from build123d import *

# Parameters (mm, degrees)
BOSS_EXTRUDE1_DEPTH     = 2
SKETCH2_R               = 3.25
CUT_HOLES_DEPTH         = 3
CUT_HOLES_DEPTH_BACK    = 3
CUT_EXTRUDE1_DEPTH      = 3
CUT_EXTRUDE1_DEPTH_BACK = 3


with BuildPart() as part:
    # Sketch1 → Boss-Extrude1 (new body, symmetric)
    with BuildSketch(Plane(origin=(0, 0, 0), x_dir=(1, 0, 0), z_dir=(0, 1, 0))):
        with BuildLine():
            Line((86.2, 39.931942102), (86.2, -39.931942102))
            ThreePointArc((86.2, -39.931942102), (0, -81.597763245), (-86.2, -39.931942102))
            Line((-86.2, -39.931942102), (-86.2, 39.931942102))
            ThreePointArc((-86.2, 39.931942102), (0, 95), (86.2, 39.931942102))
        make_face()
    extrude(amount=BOSS_EXTRUDE1_DEPTH, both=True)

    # Sketch2 → Cut-Holes (cut, two sides)
    with BuildSketch(Plane(origin=(0, 0, 0), x_dir=(1, 0, 0), z_dir=(0, 1, 0))) as cut_holes_sk:
        with Locations((-74.7, 11)):
            Circle(SKETCH2_R)
        with Locations((-74.7, -41)):
            Circle(SKETCH2_R)
        with Locations((74.7, -41)):
            Circle(SKETCH2_R)
        with Locations((74.7, 11)):
            Circle(SKETCH2_R)
        with Locations((0, -71.597763245)):
            Circle(SKETCH2_R)
        with Locations((0, 85)):
            Circle(SKETCH2_R)
        with Locations((-75.036257902, 39.931942102)):
            Circle(SKETCH2_R)
        with Locations((75.036257902, 39.931942102)):
            Circle(SKETCH2_R)
        with BuildLine():
            ThreePointArc((14.471626034, -67.259325745), (11.744315506, -70.958890218), (15.443879979, -73.686200745))
            ThreePointArc((15.443879979, -73.686200745), (40.475581865, -66.58349782), (62.936747266, -53.448409812))
            ThreePointArc((62.936747266, -53.448409812), (63.532100029, -48.890937367), (58.974627584, -48.295584605))
            ThreePointArc((58.974627584, -48.295584605), (37.92748228, -60.603766345), (14.471626034, -67.259325745))
        make_face()
        with BuildLine():
            ThreePointArc((-62.936747266, -53.448409812), (-63.532100029, -48.890937367), (-58.974627584, -48.295584605))
            ThreePointArc((-58.974627584, -48.295584605), (-37.92748228, -60.603766345), (-14.471626034, -67.259325745))
            ThreePointArc((-14.471626034, -67.259325745), (-11.744315506, -70.958890218), (-15.443879979, -73.686200745))
            ThreePointArc((-15.443879979, -73.686200745), (-40.475581865, -66.58349782), (-62.936747266, -53.448409812))
        make_face()
        with BuildLine():
            ThreePointArc((-63.94162293, 50.936542452), (-68.508644796, 50.419520904), (-69.025666344, 54.98654277))
            ThreePointArc((-69.025666344, 54.98654277), (-45.1765399, 75.809911903), (-15.512787354, 86.875865052))
            ThreePointArc((-15.512787354, 86.875865052), (-11.742100438, 84.24776304), (-14.37020245, 80.477076125))
            ThreePointArc((-14.37020245, 80.477076125), (-41.849089369, 70.226179015), (-63.94162293, 50.936542452))
        make_face()
        with BuildLine():
            ThreePointArc((15.512787354, 86.875865052), (11.742100438, 84.24776304), (14.37020245, 80.477076125))
            ThreePointArc((14.37020245, 80.477076125), (41.849089369, 70.226179015), (63.94162293, 50.936542452))
            ThreePointArc((63.94162293, 50.936542452), (68.508644796, 50.419520904), (69.025666344, 54.98654277))
            ThreePointArc((69.025666344, 54.98654277), (45.1765399, 75.809911903), (15.512787354, 86.875865052))
        make_face()
    extrude(amount=CUT_HOLES_DEPTH, mode=Mode.SUBTRACT)
    extrude(cut_holes_sk.sketch, amount=-CUT_HOLES_DEPTH_BACK, mode=Mode.SUBTRACT)

    # Sketch3 → Cut-Extrude1 (cut, two sides)
    with BuildSketch(Plane(origin=(0, 0, 0), x_dir=(1, 0, 0), z_dir=(0, 1, 0))) as cut_extrude1_sk:
        with BuildLine():
            Line((5, 1.7), (40, 1.7))
            ThreePointArc((40, 1.7), (41.7, 0), (40, -1.7))
            Line((40, -1.7), (5, -1.7))
            ThreePointArc((5, -1.7), (3.3, 0), (5, 1.7))
        make_face()
        with BuildLine():
            Line((-5, -1.7), (-40, -1.7))
            ThreePointArc((-40, -1.7), (-41.7, 0), (-40, 1.7))
            Line((-40, 1.7), (-5, 1.7))
            ThreePointArc((-5, 1.7), (-3.3, 0), (-5, -1.7))
        make_face()
        with BuildLine():
            Line((-1.7, 55), (-1.7, 10))
            ThreePointArc((-1.7, 10), (0, 8.3), (1.7, 10))
            Line((1.7, 10), (1.7, 55))
            ThreePointArc((1.7, 55), (0, 56.7), (-1.7, 55))
        make_face()
        with BuildLine():
            Line((-1.7, -55), (-1.7, -10))
            ThreePointArc((-1.7, -10), (0, -8.3), (1.7, -10))
            Line((1.7, -10), (1.7, -55))
            ThreePointArc((1.7, -55), (0, -56.7), (-1.7, -55))
        make_face()
        with BuildLine():
            ThreePointArc((-46.094214922, 33.104166667), (-46.838138391, 37.639756802), (-51.373728526, 36.895833333))
            ThreePointArc((-51.373728526, 36.895833333), (-63.25, 0), (-51.373728526, -36.895833333))
            ThreePointArc((-51.373728526, -36.895833333), (-46.838138391, -37.639756802), (-46.094214922, -33.104166667))
            ThreePointArc((-46.094214922, -33.104166667), (-56.75, 0), (-46.094214922, 33.104166667))
        make_face()
        with BuildLine():
            ThreePointArc((51.373728526, -36.895833333), (46.838138391, -37.639756802), (46.094214922, -33.104166667))
            ThreePointArc((46.094214922, -33.104166667), (56.75, 0), (46.094214922, 33.104166667))
            ThreePointArc((46.094214922, 33.104166667), (46.838138391, 37.639756802), (51.373728526, 36.895833333))
            ThreePointArc((51.373728526, 36.895833333), (63.25, 0), (51.373728526, -36.895833333))
        make_face()
    extrude(amount=CUT_EXTRUDE1_DEPTH, mode=Mode.SUBTRACT)
    extrude(cut_extrude1_sk.sketch, amount=-CUT_EXTRUDE1_DEPTH_BACK, mode=Mode.SUBTRACT)


solid = part.part
Source: CAD feature listing. Evaluate the final solid. Frame: model axes, mm. A direction names the side the tool comes from. Coordinates: 2 decimals unless noted, no trailing zeros. Loops run counter-clockwise (first coordinate to the right, second up) from the corner with the lowest first, then second, coordinate; pieces in that order, holes last. Notation, with made-up numbers: (23.5, -26.75) - (42.5, -26.75) arc R12 cw to (42.5, -8.75) - close; hole circle Ø3 at (47, 74.25). An arc over 180 degrees is marked (long way). One line per question, with ' | ' between items.
1) Section C-C, the plane y = -0.2. Give the number of separate pieces and of enclosed holes in the cut face, then the cut area to 3 significant figures.
Report:
separate pieces: 1 | enclosed holes: 18 | area: 22,100 mm²
2) Section B-B, the plane z = -69. Return loops of the section in (x, y), then the cut area to 3 significant figures.
Report:
outline: (-65.3, -2) - (-55.02, -2) - (-55.02, 2) - (-65.3, 2) - close; (-43.84, -2) - (43.84, -2) - (43.84, 2) - (-43.84, 2) - close; (55.02, -2) - (65.3, -2) - (65.3, 2) - (55.02, 2) - close | area: 433 mm²
3) Set-up query: faces 3 (the face through (1, -2, -8)), 4 (the face through (22, 0, -1.7)). Return all of +Z, -Z, +X, -X, +Y, -Y with unobstructed straight access to the full face (end or side cutting, diameter ignored); none if empty.
Report:
face 3: +Z, -Z, +X, -X, -Y | face 4: +Y, -Y
4) Pull-direction query (Z, two-part tool) for faces 1 (the face through (-86.2, 0, 1)), 2 (the face through (1.7, 0, 32)); classes: released by +Z, released by -Z, zero draft, split by the parting line, or undercut.
Report:
face 1: zero draft | face 2: undercut
5) Line query: line 1 along Z through (x, y) = (0, 1.1); line 2 along X through (y, z) = (1.45, -62); line 3 along Z through (x, y) = (37, 1.8). Output: solid intervals per line, ascending.
Report:
line 1: z = -95 to -88.25, -81.75 to -56.7, -8.3 to 8.3, 56.7 to 68.35, 74.85 to 81.6 | line 2: x = -71.98 to -62.8, -53.28 to 53.28, 62.8 to 71.98 | line 3: z = -87.5 to -80.12, -72.9 to -1.7, 1.7 to 60.99, 67.99 to 75.19
6) Section D-D, the plane z = 62.5. Return loops of the section in (x, y), then the cut area to 3 significant figures.
Report:
outline: (-61.94, -2) - (-48.96, -2) - (-48.96, 2) - (-61.94, 2) - close; (-33.13, -2) - (33.13, -2) - (33.13, 2) - (-33.13, 2) - close; (48.96, -2) - (61.94, -2) - (61.94, 2) - (48.96, 2) - close | area: 369 mm²
7) Section A-A, the plane x = 74.7. Return loops of the section in (y, z), then the cut area to 3 significant figures.
Report:
outline: (-2, -58.69) - (2, -58.69) - (2, -43.16) - (-2, -43.16) - close; (-2, -36.7) - (2, -36.7) - (2, -14.25) - (-2, -14.25) - close; (-2, -7.75) - (2, -7.75) - (2, 37.75) - (-2, 37.75) - close; (-2, 44.25) - (2, 44.25) - (2, 52.34) - (-2, 52.34) - close | area: 366 mm²
8) First-contact query: P1, Ø1, axis at x = -62, y = 1, coming from the +Z side; P2, Ø1.2, axis at x = 20, y = 0.5, coming from the -Z side; P3, Ø1, axis at y = 1, z = 55.5, coming from the +X side. Flat tips, straight axial feed; report the tip coordinate or a pass-through.
Report:
P1: stops at z = 62.8 | P2: stops at z = -93 | P3: stops at x = 71.72
